Work out the finished part from the listing and answer in its coordinate system (mm). Face numbers are marked on the shaded views. A direction names the side the tool comes from. Give positions to 0.01 mm unless a question says otherwise; leave off trailing zeros. Write each loop counter-clockwise with the first axis right and the second up, starting at its lowest first coordinate (ties: lowest second). Pieces come first, ordered by that corner, then holes. Notation, with made-up numbers: (59, -21) -> (103, -21) arc R27 ccw to (103, 13) -> close; hole circle Ø5 at (-13, -31). An arc over 180 degrees is marked (long way). Write item = value, one per line. Start each with the question number.
from build123d import *

# Parameters (mm, degrees)
FILLET1_R = 1.27


with BuildPart() as part:
    # Sketch1 → Revolve1 (revolve)
    with BuildSketch(Plane.XY):
        with BuildLine():
            Line((0, 17.78), (0, 0))
            Line((0, 0), (203.2, 0))
            Line((203.2, 0), (203.2, 12.7))
            Line((203.2, 12.7), (101.6, 12.7))
            Line((101.6, 12.7), (101.6, 17.78))
            Line((101.6, 17.78), (99.06, 17.78))
            ThreePointArc((99.06, 17.78), (97.192874103, 13.84504892), (92.964, 12.802636843))
            Line((92.964, 12.802636843), (68.58, 17.78))
            Line((68.58, 17.78), (0, 17.78))
        make_face()
    revolve(axis=Axis((-70.891441255, 0, 0), (1, 0, 0)))

    # Fillet1
    fillet1_edges = [part.edges().sort_by_distance(p)[0] for p in [
        (101.6, -12.7, 0),
    ]]
    fillet(fillet1_edges, radius=FILLET1_R)


solid = part.part
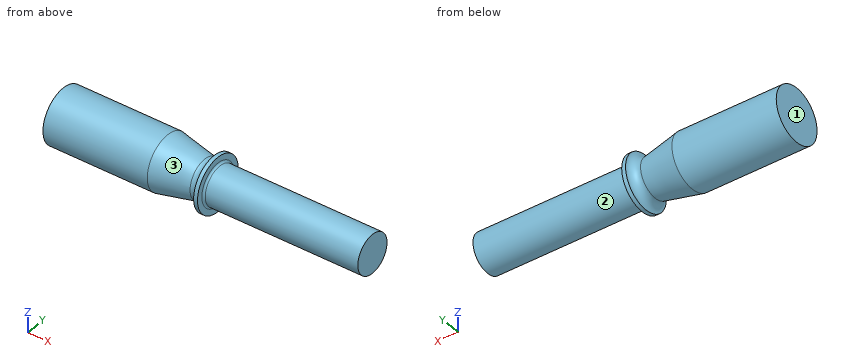
(1) Find the intervals of material crossed by line 1 along Y through (x, z) = (32, 1); line 2 along Z through (x, y) = (67.5, 7); line 3 along Y through (x, z) = (67, -5.5), in increasing order.
(2) Each of these flat-tipped pins is pushed along its axis until it touches: pin 1 (10 mm diameter, centred on x = 170.5, y = 8.5, fed in from -Z); pin 2 (4 mm diameter, centred on x = 158, y = 9.5, fed in from -Z); pin 3 (12 mm diameter, centred on x = 64.5, y = -5.5, fed in from +Z); pin 4 (2 mm diameter, centred on x = 80, z = -0.5, fed in from -Y). Where does it stop, or does it pass through?
(3) A cutting plane is placed at C-C, the plane x = 177. Write down the section's boundary in (y, z).
(4) For the marked faces 1, 2 and 3, determine the directions among +Z, -Z, +X, -X, +Y, -Y from which every point of the face is accessible in a straight line to the end or side of a thin tool.
(5) A cutting plane is placed at A-A, the plane y = 0. Write down the section's boundary in (x, z), then the cut area to 3 significant figures.
Results list:
q1.line_1 = -17.75 to 17.75
q1.line_2 = -16.34 to 16.34
q1.line_3 = -16.91 to 16.91
q2.pin_1 = -12.21
q2.pin_2 = -10.25
q2.pin_3 = 17.78
q2.pin_4 = -15.65
q3.outline = circle Ø25.4 at (0, 0)
q4.face_1 = +Z, -Z, -X, +Y, -Y
q4.face_2 = +X
q4.face_3 = none
q5.outline = (0, -17.78) -> (68.58, -17.78) -> (92.96, -12.8) arc R5.08 cw to (99.06, -17.78) -> (101.6, -17.78) -> (101.6, -13.97) arc R1.27 cw to (102.87, -12.7) -> (203.2, -12.7) -> (203.2, 12.7) -> (102.87, 12.7) arc R1.27 cw to (101.6, 13.97) -> (101.6, 17.78) -> (99.06, 17.78) arc R5.08 cw to (92.96, 12.8) -> (68.58, 17.78) -> (0, 17.78) -> close
q5.area = 6,020 mm²
